from build123d import *

# Parameters (mm, degrees)
SKETCH_R         = 4.6
PAD_DEPTH        = 6.4
SKETCH001_R      = 3.175
PAD001_DEPTH     = 19
CHAMFER_SIZE     = 1.5
FILLET_R         = 1.2
SKETCH002_R      = 1.725
POCKET_DEPTH     = 11
FILLET001_R      = 0.5
SKETCH004_R      = 1.8
POCKET001_DEPTH  = 5
POCKET002_DEPTH  = 5
SKETCH006_R      = 1.7
POCKET003_DEPTH  = 5
CHAMFER001_SIZE2 = 0.5
CHAMFER001_SIZE  = 0.7


with BuildPart() as part:
    # Sketch → Pad (new body)
    with BuildSketch(Plane.XY):
        Circle(SKETCH_R)
    extrude(amount=PAD_DEPTH)

    # Sketch001 (on Face3 of Pad) → Pad001 (join)
    with BuildSketch(Plane.XY.offset(6.4)):
        Circle(SKETCH001_R)
    extrude(amount=PAD001_DEPTH)

    # Chamfer
    chamfer_edges = [part.edges().sort_by_distance(p)[0] for p in [
        (-3.175, 0, 25.4),
    ]]
    chamfer(chamfer_edges, length=CHAMFER_SIZE)

    # Fillet
    fillet_edges = [part.edges().sort_by_distance(p)[0] for p in [
        (-4.6, 0, 0),
    ]]
    fillet(fillet_edges, radius=FILLET_R)

    # Sketch002 (on Face4 of Fillet) → Pocket (cut)
    with BuildSketch(Plane(origin=(0, 0, 0), x_dir=(1, 0, 0), z_dir=(0, 0, -1))):
        Circle(SKETCH002_R)
    extrude(amount=-POCKET_DEPTH, mode=Mode.SUBTRACT)

    # Fillet001
    fillet001_edges = [part.edges().sort_by_distance(p)[0] for p in [
        (-1.725, 0, 0),
    ]]
    fillet(fillet001_edges, radius=FILLET001_R)

    # Sketch003 → Groove (revolve, cut)
    with BuildSketch(Plane.XZ):
        with BuildLine():
            ThreePointArc((3, 16.4), (2.3, 15.7), (3, 15))
            Line((3, 15), (4.410793, 15))
            Line((4.410793, 16.4), (4.410793, 15))
            Line((3, 16.4), (4.410793, 16.4))
        make_face()
    revolve(axis=Axis((0, 0, 0), (0, 0, 1)), mode=Mode.SUBTRACT)

    # Sketch004 → Pocket001 (cut)
    with BuildSketch(Plane.XZ):
        with Locations((0, 3.5)):
            Circle(SKETCH004_R)
    extrude(amount=-POCKET001_DEPTH, mode=Mode.SUBTRACT)

    # Sketch005 → Pocket002 (cut)
    with BuildSketch(Plane.YZ.offset(-2.9)):
        with BuildLine():
            ThreePointArc((1.2, 7.7), (0, 8.9), (-1.2, 7.7))
            Line((-1.2, 7.7), (-1.2, 3.7))
            ThreePointArc((-1.2, 3.7), (0, 2.5), (1.2, 3.7))
            Line((1.2, 7.7), (1.2, 3.7))
        make_face()
    extrude(amount=-POCKET002_DEPTH, mode=Mode.SUBTRACT)

    # Sketch006 → Pocket003 (cut)
    with BuildSketch(Plane(origin=(0, 0, 0), x_dir=(0.707107, 0.707107, 0), z_dir=(0.707107, -0.707107, 0))):
        with Locations((0, 3.5)):
            Circle(SKETCH006_R)
    extrude(amount=POCKET003_DEPTH, mode=Mode.SUBTRACT)

    # Chamfer001
    chamfer001_edges = [part.edges().sort_by_distance(p)[0] for p in [
        (1.820335, -4.224498, 3.5),
        (-1.8, 4.233202, 3.5),
    ]]
    chamfer001_side = part.faces().sort_by_distance((-4.6, 0, 1.340114))[0]
    chamfer(chamfer001_edges, length=CHAMFER001_SIZE, length2=CHAMFER001_SIZE2, reference=chamfer001_side)


solid = part.part
Model file for the job. Use its own axes, mm. A direction names the side the tool comes from. Round coordinates to 2 decimals unless told otherwise and drop trailing zeros. Order: outer loops, then holes, each group sorted by start corner. A loop starts at its lowest first (then second) coordinate and runs counter-clockwise, first axis right, second up. Notation, with made-up numbers: M -2,31 L 21,31 A19 cw 21,47 Z; hole C 25,-20.5 d9. An arc over 180 degrees is marked long. Write each question's results on one line, items separated by ' | '. Start each with the question number.
(1) Drop flat-ended pins along their axis: pin 1 (4 mm diameter, centred on x = -0.5, z = 12.5, fed in from -Y) (3 decimals); pin 2 (2 mm diameter, centred on x = -1, y = -2, fed in from +Z); pin 3 (5 mm diameter, centred on y = -0.5, z = 13, fed in from +X) (3 decimals); pin 4 (4 mm diameter, centred on x = 1.5, z = 11, fed in from +Y) (3 decimals). Give the stop position or say it passes through.
(2) Saw through at A-A, the plane z = 11.25. Give the cut face in (x, y) (3 decimals).
(3) Which spindle directions (+Z, -Z, +X, -X, +Y, -Y) get a long thin tool onto all of the face, cutting with end or side? Do faces 5 (the face through (-2.9, 0, 6)), 6 (the face through (-1.8, 2.48, 3.58)), 7 (the face through (3.03, 0.95, 10.64)), 8 (the face through (0, 0, 11)). Say none if no direction does.
(4) Probe probe 1 along Y at (x, z) = (0, 8.5) (3 decimals); probe 2 along X at (y, z) = (0, 5.5) (3 decimals); probe 3 along X at (y, z) = (0.95, 3.5). List the from-to ranges inside material, lowest first. Write a range as from..to.
(5) Two-plate mould, pull along Y, no slides. Class faces 1 (the face through (-3.7, 0, 2.5)), 2 (the face through (3, -2, 6.4)), 3 (the face through (-0.69, -3.1, 20.1)), 4 (the face through (-1.27, -1.17, 5.68)): pulls with the +Y half, pulls with the -Y half, needs draft (parallel to the pull), parting line crosses it, or undercut.
Established:
1) pin 1: stops at y = -3.175 | pin 2: stops at z = 25.4 | pin 3: stops at x = 3.175 | pin 4: stops at y = 3.175
2) outline: C 0,0 d6.35
3) face 5: -X | face 6: +Y | face 7: +Z | face 8: -Z
4) probe 1: y = -3.175..-1.725, 1.725..3.175 | probe 2: x = -2.9..-1.725, 1.725..4.6 | probe 3: x = -2.9..-1.8, 1.8..4.5
5) face 1: undercut | face 2: needs draft | face 3: parting line crosses it | face 4: undercut
